Part model, mm, in its own coordinate system. Face numbers are marked on the shaded views. A direction names the side the tool comes from. Coordinates: 2 decimals unless noted, no trailing zeros. Loops run counter-clockwise (first coordinate to the right, second up) from the corner with the lowest first, then second, coordinate; pieces in that order, holes last. Notation, with made-up numbers: (-8.5, -21.5) -> (37.5, -21.5) arc R33 ccw to (37.5, 13.5) -> close; hole circle Ø6 at (-21, -25.5). An arc over 180 degrees is marked (long way). One line per question, with ' | ' between items. Start each with the question number.
1) Drop flat-ended pins along their axis: pin 1 (1.2 mm diameter, centred on y = 1.5, z = 3, fed in from +X); pin 2 (2 mm diameter, centred on x = 4.5, z = 1.5, fed in from -Y); pin 3 (0.6 mm diameter, centred on x = -2.5, y = -1.5, fed in from +Z). Give the stop position or say it passes through.
2) Cut at D-D (z = 4.5). List the corners of the cut face in (x, y), plus the area to 3 significant figures.
3) Probe L1, parallel to Y at x = 0, z = 5.9; L2, parallel to Z at x = -2, y = 2.75; L3, parallel to Y at x = -1.75, z = 1.5. List the from-to ranges inside material, lowest first. Write a range as from..to.
4) Two-plate mould, pull along Y, no slides. Class the marked faces 1, 2 and 3: released by +Y, released by -Y, zero draft, split by the parting line, or undercut.
5) Cut at B-B (y = 0). List the corners of the cut face in (x, z).
6) 3-axis set-ups, long thin cutter, end or side, ignore diameter. For the marked faces 4, 5 and 6: which of +Z, -Z, +X, -X, +Y, -Y reach the whole face in a straight line?
7) Cut at C-C (x = 0). List the corners of the cut face in (y, z).
8) Cut at A-A (z = 3.75). List the corners of the cut face in (x, y) (3 decimals).
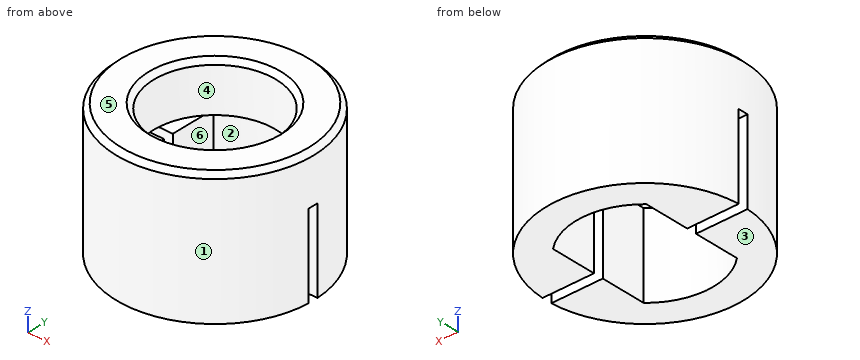
Autodesk Inventor part; units mm, degrees
ref_plane "Work Plane1" through (-2.375, -3.5, 4.25) normal (0, 0, 1) x (1, 0, 0)
ref_plane "YZ Plane" through (0, 0, 0) normal (1, 0, 0) x (0, 1, 0)
ref_plane "XZ Plane" through (0, 0, 0) normal (0, 1, 0) x (-1, 0, 0)
sketch "Sketch1" plane through (0, 0, 0) normal (0, 0, 1) x (1, 0, 0)
  line L0 (-2.375, 2.5709) -> (-2.375, -2.5709)
  arc A0 (-2.375, -2.5709) -> (2.375, -2.5709) centre (0, 0) ccw
  line L1 (2.375, -2.5709) -> (2.375, 2.5709)
  arc A1 (2.375, 2.5709) -> (-2.375, 2.5709) centre (0, 0) ccw
  circle A2 centre (0, 0) radius 0.875
  circle A3 centre (0, 0) radius 5
  dimension "d0" = 10
ref_plane "Work Plane1" through (-2.375, -3.5, 4.25) normal (0, 0, 1) x (1, 0, 0)
extrude "Extrusion1" add sketch "Sketch1" along normal up to surface (4.25 mm away) contours A3
sketch "Sketch2" plane through (0, 0, 4.25) normal (0, 0, 1) x (1, 0, 0)
  circle A0 centre (0, 0) radius 3.1
  circle A1 centre (0, 0) radius 5
  dimension "d3" = 6.2
extrude "Extrusion2" add sketch "Sketch2" along normal blind 2.5
sketch "Sketch3" plane through (0, 0, 0) normal (0, 0, -1) x (-1, 0, 0)
  line L0 (-5.064, 0) -> (5.064, 0) construction
  line L1 (-5.064, -0.25) -> (5.064, -0.25)
  line L2 (5.064, 0.25) -> (-5.064, 0.25)
  arc A0 (-5.064, 0.25) -> (-5.064, -0.25) centre (-5.064, 0) ccw
  arc A1 (5.064, -0.25) -> (5.064, 0.25) centre (5.064, 0) ccw
  point P0 (0, 0)
  dimension "d6" = 0.5
extrude "Extrusion3" cut sketch "Sketch3" against normal blind 4.25
chamfer "Chamfer1" distance 0.25 angle 45 2 edges at (-3.1, 0, 6.75) (-5, 0, 6.75)
properties part number "MagnetHolder"
Reported:
1) pin 1: stops at x = 4.92 | pin 2: stops at y = -3.57 | pin 3: stops at z = 6.62
2) outline: circle Ø10 at (0, 0); hole circle Ø6.2 at (0, 0) | area: 48.3 mm²
3) L1: y = -5..-3.1, 3.1..5 | L2: z = 4.25..6.75 | L3: y = -4.68..-3.03, 3.03..4.68
4) face 1: split by the parting line | face 2: undercut | face 3: zero draft
5) outline: (-5, 4.25) -> (-3.1, 4.25) -> (-3.1, 6.5) -> (-3.35, 6.75) -> (-4.75, 6.75) -> (-5, 6.5) -> close; (3.1, 4.25) -> (5, 4.25) -> (5, 6.5) -> (4.75, 6.75) -> (3.35, 6.75) -> (3.1, 6.5) -> close
6) face 4: +Z | face 5: +Z, +X, -X, +Y, -Y | face 6: -Z
7) outline: (-5, 0) -> (-3.5, 0) -> (-3.5, 4.25) -> (-3.1, 4.25) -> (-3.1, 6.5) -> (-3.35, 6.75) -> (-4.75, 6.75) -> (-5, 6.5) -> close; (3.1, 4.25) -> (3.5, 4.25) -> (3.5, 0) -> (5, 0) -> (5, 6.5) -> (4.75, 6.75) -> (3.35, 6.75) -> (3.1, 6.5) -> close
8) outline: (-4.994, -0.25) arc R5 ccw to (4.994, -0.25) -> (2.375, -0.25) -> (2.375, -2.571) arc R3.5 cw to (-2.375, -2.571) -> (-2.375, -0.25) -> close; (-4.994, 0.25) -> (-2.375, 0.25) -> (-2.375, 2.571) arc R3.5 cw to (2.375, 2.571) -> (2.375, 0.25) -> (4.994, 0.25) arc R5 ccw to start
